```python
from build123d import *

# Parameters (mm, degrees)
SKETCH2_W           = 100
SKETCH2_H           = 105
BOSS_EXTRUDE1_DEPTH = 10
SKETCH5_R           = 15
SKETCH5_R_2         = 5
CUT_EXTRUDE1_DEPTH  = 10
CUT_EXTRUDE2_REACH  = 12
SKETCH6_W           = 22.5
SKETCH6_H           = 12.5
FILLET2_R           = 0.5
SKETCH12_R          = 4
CUT_EXTRUDE3_DEPTH  = 10
SKETCH13_W          = 4
SKETCH13_H          = 12.5
BOSS_EXTRUDE2_DEPTH = 3
FILLET3_R           = 2
CUT_EXTRUDE6_REACH  = 18.794
SKETCH14_W          = 154.448813283
SKETCH14_H          = 123.004866117
SKETCH14_W_2        = 99.5
SKETCH14_H_2        = 104.5


with BuildPart() as part:
    # Sketch2 → Boss-Extrude1 (new body)
    with BuildSketch(Plane(origin=(0, 0, 0), x_dir=(1, 0, 0), z_dir=(0, 1, 0))):
        Rectangle(SKETCH2_W, SKETCH2_H)
    extrude(amount=BOSS_EXTRUDE1_DEPTH)

    # Sketch5 → Cut-Extrude1 (cut)
    with BuildSketch(Plane.XZ):
        with Locations((-15.347413929, 31.5)):
            Circle(SKETCH5_R)
        with Locations((-40, 0)):
            Circle(SKETCH5_R_2)
    cut_extrude1 = extrude(amount=-CUT_EXTRUDE1_DEPTH, mode=Mode.SUBTRACT)

    # Mirror1: Cut-Extrude1 across plane
    add(cut_extrude1.mirror(Plane.XY), mode=Mode.SUBTRACT)

    # Sketch6 → Cut-Extrude2 (cut, up to next)
    with BuildSketch(Plane.XZ, mode=Mode.PRIVATE) as cut_extrude2_sk1:
        with Locations((-34.75, 0)):
            Rectangle(SKETCH6_W, SKETCH6_H)
    cut_extrude2_tool1 = extrude(cut_extrude2_sk1.sketch, amount=-CUT_EXTRUDE2_REACH, mode=Mode.PRIVATE) & part.part
    add(cut_extrude2_tool1.solids().sort_by_distance((-34.75, 0, 0))[0], mode=Mode.SUBTRACT)

    # Sweep1: sweep along a path in Sketch11
    with BuildLine(Plane(origin=(7.914589695, 0, 7.643030426), x_dir=(0, -1, 0), z_dir=(0.7193398, 0, 0.69465837))) as sweep1_path:
        Line((0, -49.687749169), (6.793793585, -43.105226771))
    # Sketch7 → Sweep1 (sweep)
    with BuildSketch(Plane.XZ):
        with BuildLine():
            ThreePointArc((-6.352107338, 43.503518623), (-25.0878405, 42.907194669), (-28.61191488, 24.496214272))
            ThreePointArc((-28.61191488, 24.496214272), (-28.155696018, 46.500017309), (-6.352107338, 43.503518623))
        make_face()
    sweep(path=sweep1_path.line)

    # Fillet2
    fillet2_edges = [part.edges().sort_by_distance(p)[0] for p in [
        (-20.515236217, -6.793793585, 38.172124321),
        (-26.325612738, -3.396896793, 22.128679098),
        (-4.065805196, -3.396896793, 41.135983449),
    ]]
    fillet(fillet2_edges, radius=FILLET2_R)

    # Sketch12 → Cut-Extrude3 (cut)
    with BuildSketch(Plane(origin=(0, 10, 0), x_dir=(1, 0, 0), z_dir=(0, 1, 0))):
        with Locations((42, 44.5)):
            Circle(SKETCH12_R)
    cut_extrude3 = extrude(amount=-CUT_EXTRUDE3_DEPTH, mode=Mode.SUBTRACT)

    # Mirror2: Cut-Extrude3 across plane
    add(cut_extrude3.mirror(Plane.XY), mode=Mode.SUBTRACT)

    # Sketch13 → Boss-Extrude2 (add)
    with BuildSketch(Plane(origin=(0, 10, 0), x_dir=(1, 0, 0), z_dir=(0, 1, 0))):
        with Locations((-48, 0)):
            Rectangle(SKETCH13_W, SKETCH13_H)
        with Locations((-21.5, 0)):
            Rectangle(SKETCH13_W, SKETCH13_H)
    extrude(amount=BOSS_EXTRUDE2_DEPTH)

    # Fillet3
    fillet3_edges = [part.edges().sort_by_distance(p)[0] for p in [
        (-19.5, 11.5, 6.25),
        (-19.5, 11.5, -6.25),
    ]]
    fillet(fillet3_edges, radius=FILLET3_R)

    # Sketch14 → Cut-Extrude6 (cut, up to next)
    with BuildSketch(Plane(origin=(0, 10, 0), x_dir=(1, 0, 0), z_dir=(0, 1, 0)), mode=Mode.PRIVATE) as cut_extrude6_sk1:
        with Locations((-5.953267194, 1.602475316)):
            Rectangle(SKETCH14_W, SKETCH14_H)
        Rectangle(SKETCH14_W_2, SKETCH14_H_2, mode=Mode.SUBTRACT)
    cut_extrude6_tool1 = extrude(cut_extrude6_sk1.sketch, amount=-CUT_EXTRUDE6_REACH, mode=Mode.PRIVATE) & part.part
    add(cut_extrude6_tool1.solids().sort_by_distance((-5.953267, 10, -61.130456))[0], mode=Mode.SUBTRACT)


solid = part.part
```
Geometry: final body of the model. Coordinates: model frame, mm. A direction names the side the tool comes from. Coordinates: 2 decimals unless noted, no trailing zeros. Write each loop counter-clockwise with the first axis right and the second up, starting at its lowest first coordinate (ties: lowest second). Pieces come first, ordered by that corner, then holes. Notation, with made-up numbers: M 11,18.5 L 32,18.5 A21 ccw 32,43.5 Z; hole C 34.5,63.25 d2. An arc over 180 degrees is marked long. Answer as CSV lines item,"result". Start each with the question number.
Q1. Cut plane C-C on z = -44.5. Return the cut outline in (x, y).
Q2. Reachability of faces 1 (the flat face through (-19.5, 11, 0)), 2 (the flat face through (-23.5, 6, 0)), 3 (the flat face through (-48, 11, -6.25)), 4 (the flat face through (-50, 11, 0)), 5 (the flat face through (-21, -6.794, 40)) from +Z, -Z, +X, -X, +Y, -Y: full face, straight path, thin tool, end or side. Return the list, or none.
Q3. Pin query (flat end, axial travel): P1, Ø8, axis at y = 3.5, z = -20.5, coming from the -X side; P2, Ø6.5, axis at x = 42, z = -44.5, coming from the +Y side; P3, Ø3, axis at x = 8.5, z = -5.5, coming from the +Y side; P4, Ø8, axis at x = 37, z = 5.5, coming from the -Y side. Return the tip coordinate at first contact, or that it passes through.
Q4. Line query: line 1 (Z direction, x = 42, y = 6.5); line 2 (X direction, y = 1.5, z = -0.5); line 3 (Z direction, x = -5.5, y = 8.25). Output: solid intervals per line, ascending. Write a range as from..to.
Q5. Cut plane B-B on z = -31.5. Return the cut outline in (x, y).
Q6. Mould query, pull axis Z, two halves, no side actions, for faces 6 (the flat face through (-22, 13, 0)), 7 (the flat face through (-1, 5, 52.25)), 8 (the cylindrical face through (38.8, 5.1, 42.1)). Classes: released by +Z, released by -Z, zero draft, split by the parting line, or undercut.
Q7. Cut plane A-A on x = -43. Return the cut outline in (y, z).
Q8. Cut plane D-D on x = 29.5. Return the cut outline in (y, z), then the cut area to 4 significant figures.
Findings below:
1,outline,"M -49.75,0 L -22.83,0 L -22.83,10 L -49.75,10 Z; M -7.86,0 L 38,0 L 38,10 L -7.86,10 Z; M 46,0 L 49.75,0 L 49.75,10 L 46,10 Z"
2,face 1,"+Z, -Z, +X, +Y"
2,face 2,"+Y, -Y"
2,face 3,"-Z, +X, -X, +Y"
2,face 4,"+Z, -Z, -X, +Y, -Y"
2,face 5,"+Z, -Z, +X, -X, -Y"
3,P1,"stops at x = -49.75"
3,P2,"passes through"
3,P3,"stops at y = 10"
3,P4,"stops at y = 0"
4,line 1,"z = -52.25..-48.5, -40.5..40.5, 48.5..52.25"
4,line 2,"x = -49.75..-46, -23.5..49.75"
4,line 3,"z = -52.25..-42.81, -20.19..20.19, 42.81..52.25"
5,outline,"M -49.75,0 L -30.35,0 L -30.35,10 L -49.75,10 Z; M -0.35,0 L 49.75,0 L 49.75,10 L -0.35,10 Z"
6,face 6,"zero draft"
6,face 7,"released by +Z"
6,face 8,"undercut"
7,outline,"M 0,-52.25 L 10,-52.25 L 10,-6.25 L 0,-6.25 Z; M 0,6.25 L 10,6.25 L 10,52.25 L 0,52.25 Z"
8,outline,"M 0,-52.25 L 10,-52.25 L 10,52.25 L 0,52.25 Z"
8,area,"1,045 mm2"
